from build123d import *

# Parameters (mm, degrees)
F0_W      = 129
F0_H      = 143.5
F0_W_2    = 125
F0_H_2    = 139.5
F1_DEPTH  = 3
F2_DEPTH  = 2
F3_SIZE   = 1.99999
F5_DEPTH  = 25
F6_W      = 125
F6_H      = 141.5
F6_W_2    = 124.5
F6_H_2    = 139
F6_W_3    = 122.5
F6_H_3    = 137
F7_DEPTH  = 1
F8_DEPTH  = 3
F9_SIZE   = 1.99999
F10_DEPTH = 2
F10_TAPER = 45


# Not quite as in the source:
# - a fillet or chamfer is up to 0.001 mm smaller than in the source, because OpenCascade refuses the exact size
# - a feature names something its author has since deleted; it is built from what else it names


with BuildPart() as f1:
    # F0 (on Top) → F1 (new body)
    with BuildSketch(Plane.XY):
        Rectangle(F0_W, F0_H)
        Rectangle(F0_W_2, F0_H_2, mode=Mode.SUBTRACT)
        Rectangle(F0_W_2, F0_H_2)
    extrude(amount=F1_DEPTH)

    # F0 (on Top) → F2 (cut)
    with BuildSketch(Plane.XY):
        Rectangle(F0_W_2, F0_H_2)
    extrude(amount=F2_DEPTH, mode=Mode.SUBTRACT)

    # F3 (size 2 in the source; OpenCascade refuses exactly that, so slightly less here)
    f3_edges = [f1.edges().sort_by_distance(p)[0] for p in [
        (0, -69.75, 2),
        (62.5, 0, 2),
        (0, 69.75, 2),
        (-62.5, 0, 2),
    ]]
    chamfer(f3_edges, length=F3_SIZE)

    # F4 (on face) → F5 (join)
    with BuildSketch(Plane.XY.offset(3)):
        Polygon((-64.5, 71.75), (-64.5, -71.75), (-62.5, -71.75), (-62.5, 69.75), (62.5, 69.75), (62.5, -71.75), (64.5, -71.75), (64.5, 71.75), align=None)
    extrude(amount=F5_DEPTH)

    # F6 (on face) → F7 (join)
    with BuildSketch(Plane.XY.offset(28)):
        with Locations((0, -1)):
            Rectangle(F6_W, F6_H)
        Rectangle(F6_W_2, F6_H_2, mode=Mode.SUBTRACT)
        Rectangle(F6_W_2, F6_H_2)
        Rectangle(F6_W_3, F6_H_3, mode=Mode.SUBTRACT)
        Rectangle(F6_W_3, F6_H_3)
        Polygon((-64.5, 71.75), (-64.5, -71.75), (-62.5, -71.75), (-62.5, 69.75), (62.5, 69.75), (62.5, -71.75), (64.5, -71.75), (64.5, 71.75), align=None)
    extrude(amount=F7_DEPTH)

    # F6 (on face) → F8 (join)
    with BuildSketch(Plane.XY.offset(28)):
        Rectangle(F6_W_2, F6_H_2)
        Rectangle(F6_W_3, F6_H_3, mode=Mode.SUBTRACT)
        Rectangle(F6_W_3, F6_H_3)
    extrude(amount=F8_DEPTH)

    # F9 (size 2 in the source; OpenCascade refuses exactly that, so slightly less here)
    f9_edges = [f1.edges().sort_by_distance(p)[0] for p in [
        (-62.25, 0, 31),
        (0, 69.5, 31),
        (0, -69.5, 31),
        (62.25, 0, 31),
    ]]
    chamfer(f9_edges, length=F9_SIZE)

    # F6 (on face) → F10 (cut)
    with BuildSketch(Plane.XY.offset(28)):
        Rectangle(F6_W_3, F6_H_3)
    extrude(amount=F10_DEPTH, taper=F10_TAPER, mode=Mode.SUBTRACT)


solid = f1.part
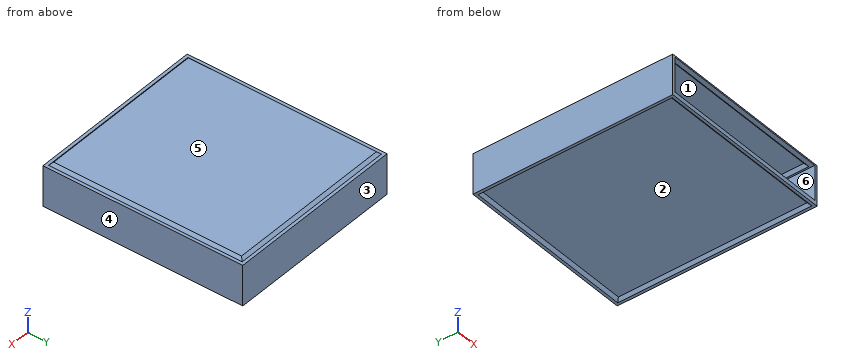
Geometry check sheet. Reference: the model listing, model coordinates, mm. Face numbers are marked on the shaded views. A direction names the side the tool comes from. Give positions to 0.01 mm unless a question says otherwise; leave off trailing zeros. Loops run counter-clockwise (first coordinate to the right, second up) from the corner with the lowest first, then second, coordinate; pieces in that order, holes last.
(1) Set-up check for the marked faces 1, 2 and 3: record each of +Z, -Z, +X, -X, +Y, -Y from which the full face is reachable in a straight line by a thin tool's end or side.
From the geometry:
face 1: none
face 2: -Z
face 3: +Z, -Z, +X, -X, +Y
(2) Release check for a two-part mould opening along Z. For the marked faces 4, 5 and 6 record: released by +Z, released by -Z, zero draft, split by the parting line, or undercut.
From the geometry:
face 4: zero draft
face 5: released by +Z
face 6: undercut
(3) Depth check by flat-ended pin: pin 1 Ø8 at (x, y) = (-19, -18.5) entering from -Z; pin 2 Ø6 at (x, z) = (4.5, 16) entering from -Y. Enter the tip coordinate at first touch or a pass-through.
From the geometry:
pin 1: stops at z = 2
pin 2: stops at y = 69.75
(4) Thickness scan on L1, parallel to X at y = -52, z = 22; L2, parallel to Z at x = -2, y = 56.5; L3, parallel to Y at x = 46.5, z = 21.5. Record the ranges inside material, lowest first.
From the geometry:
L1: x = -64.5 to -62.5, 62.5 to 64.5
L2: z = 2 to 3, 30 to 31
L3: y = 69.75 to 71.75
(5) Section check B-B on z = 15.5. Record the cut outline in (x, y).
From the geometry:
outline: (-64.5, -71.75) - (-62.5, -71.75) - (-62.5, 69.75) - (62.5, 69.75) - (62.5, -71.75) - (64.5, -71.75) - (64.5, 71.75) - (-64.5, 71.75) - close
